Geometry: final body of the model. Coordinates: model frame, mm. A direction names the side the tool comes from. Round coordinates to 2 decimals unless told otherwise and drop trailing zeros. Write each loop counter-clockwise with the first axis right and the second up, starting at its lowest first coordinate (ties: lowest second). Pieces come first, ordered by that corner, then holes. Notation, with made-up numbers: M 14,69.25 L 34,69.25 A26 ccw 34,106.25 Z; hole C 40.25,-3 d3. An arc over 180 degrees is marked long. Answer as CSV lines item,"result". Start each with the question number.
Q1. First-contact query: pin 1 (1 mm diameter, centred on y = 1.5, z = 15.5, fed in from +X); pin 2 (2 mm diameter, centred on y = 3.5, z = 3, fed in from +X); pin 3 (6 mm diameter, centred on x = -30, z = 13, fed in from -Y). Flat tips, straight axial feed; report the tip coordinate or a pass-through.
Q2. Reachability of faces 1 (the flat face through (-8.507, 1.148, 4.405)), 2 (the flat face through (-7.088, 4.317, 13.477)), 3 (the flat face through (-7.07, 1.148, 12.973)) from +Z, -Z, +X, -X, +Y, -Y: full face, straight path, thin tool, end or side. Return the list, or none.
Q3. Section query C-C on y = -1.5. Output: boundary loops of the cut face in (x, z).
Q4. Section query A-A on x = -28.5. Output: boundary loops of the cut face in (y, z).
Q5. Section query B-B on y = 7.25. Output: boundary loops of the cut face in (x, z), and give its area (3 significant figures).
Q6. Ray query, probe 1 along Y at (x, z) = (-50.5, 15.25); probe 2 along X at (y, z) = (0.75, 11.75); probe 3 along Z at (x, y) = (-79, -1.5). Return the intervals inside material, ascending.
```python
from build123d import *

# Parameters (mm, degrees)
BOSS_EXTRUDE2_DEPTH      = 5.6
CHAMFER2_SIZE            = 2.328478482
CHAMFER2_SIZE_2          = 8.69
CHAMFER3_SIZE            = 8.69
CHAMFER3_SIZE_2          = 2.328478482
CHAMFER4_SIZE            = 8.69
CHAMFER4_SIZE_2          = 2.328478482
CHAMFER5_SIZE            = 8.69
CHAMFER5_SIZE_2          = 2.328478482
FILLET1_R                = 1
SKETCH8_R                = 6.42
BOSS_EXTRUDE3_DEPTH      = 58
FILLET2_R                = 3
CUT_EXTRUDE12_DEPTH      = 16
CUT_EXTRUDE13_DEPTH      = 119.774223563
CUT_EXTRUDE13_DEPTH_BACK = 119.774223563
SKETCH19_W               = 4.551969905
SKETCH19_H               = 31.016999287


with BuildPart() as part:
    # Sketch3 → Boss-Extrude2 (new body)
    with BuildSketch(Plane(origin=(0, 0, 0), x_dir=(1, 0, 0), z_dir=(0, 1, 0))):
        with BuildLine():
            Line((-55.958218902, 0), (34.866239796, 0))
            ThreePointArc((34.866239796, 0), (43.555159042, -8.688919246), (34.866239796, -17.377838493))
            Line((34.866239796, -17.377838493), (-55.633760204, -17.377838493))
            Line((-55.633760204, -17.377838493), (-59.133760204, -14.977838493))
            Line((-59.133760204, -14.977838493), (-59.132241437, -8.577838493))
            Line((-59.132241437, -8.577838493), (-59.132241437, -2.173298587))
            Line((-59.132241437, -2.173298587), (-55.958218902, 0))
        make_face()
    extrude(amount=BOSS_EXTRUDE2_DEPTH)

    # Chamfer2
    # the kernel refuses this chamfer: 8.69, 2.328478482 mm, written as the material it takes off along each edge
    with BuildSketch(Plane(origin=(57.431750241, 5.6, 17.377838493), x_dir=(0, -0.9905000388259545, 0.13751244702128881), z_dir=(-1, 0, 0))) as chamfer2_piece_1:
        Polygon((CHAMFER2_SIZE * 0.990500038922, -CHAMFER2_SIZE * 0.137512447035), (-CHAMFER2_SIZE_2 * 0.137512447021, -CHAMFER2_SIZE_2 * 0.990500038826), (0, 0), align=None)
    extrude(amount=135.63102089, mode=Mode.SUBTRACT)

    # Chamfer3
    # the kernel refuses this chamfer: 8.69, 2.328478482 mm, written as the material it takes off along each edge
    with BuildSketch(Plane(origin=(57.431750241, 0, 17.377838493), x_dir=(0, -0.009967146577156423, -0.9999503267608394), z_dir=(-1, 0, 0))) as chamfer3_piece_1:
        Polygon((CHAMFER3_SIZE * 0.999950326761, -CHAMFER3_SIZE * 0.00996714657716), (-CHAMFER3_SIZE_2 * 0.00996714657813, -CHAMFER3_SIZE_2 * 0.999950326858), (0, 0), align=None)
    extrude(amount=135.63102089, mode=Mode.SUBTRACT)

    # Chamfer4
    # the kernel refuses this chamfer: 8.69, 2.328478482 mm, written as the material it takes off along each edge
    with BuildSketch(Plane(origin=(-78.523729347, 5.6, 0), x_dir=(0, 0.00996714657715643, 0.9999503267608394), z_dir=(1, 0, 0))) as chamfer4_piece_1:
        Polygon((CHAMFER4_SIZE * 0.999950326761, CHAMFER4_SIZE * 0.00996714657716), (-CHAMFER4_SIZE_2 * 0.00996714657813, CHAMFER4_SIZE_2 * 0.999950326858), (0, 0), align=None)
    extrude(amount=135.955479588, mode=Mode.SUBTRACT)

    # Chamfer5
    # the kernel refuses this chamfer: 8.69, 2.328478482 mm, written as the material it takes off along each edge
    with BuildSketch(Plane(origin=(-78.523729347, 0, 0), x_dir=(0, -0.009967146577156423, 0.9999503267608394), z_dir=(1, 0, 0))) as chamfer5_piece_1:
        Polygon((CHAMFER5_SIZE * 0.999950326761, -CHAMFER5_SIZE * 0.00996714657716), (-CHAMFER5_SIZE_2 * 0.00996714657813, -CHAMFER5_SIZE_2 * 0.999950326858), (0, 0), align=None)
    extrude(amount=135.955479588, mode=Mode.SUBTRACT)

    # Fillet1
    fillet1_edges = [part.edges().sort_by_distance(p)[0] for p in [
        (-55.633760204, 2.8, 17.377838493),
    ]]
    fillet(fillet1_edges, radius=FILLET1_R)

    # Sketch8 → Boss-Extrude3 (add)
    with BuildSketch(Plane(origin=(-59.130202523, 0, -0.014032034), x_dir=(-0.00023730738394525297, 0, 0.9999999718426024), z_dir=(-0.9999999718426024, 0, -0.00023730738394525297))):
        with Locations(Location((8.591870769, 2.8, 0), (0, 0, 183.840787638))):
            Circle(SKETCH8_R)
    extrude(amount=BOSS_EXTRUDE3_DEPTH)

    # Fillet2
    fillet2_edges = [part.edges().sort_by_distance(p)[0] for p in [
        (-7.788554378, 5.599710413, 8.688919246),
    ]]
    fillet(fillet2_edges, radius=FILLET2_R)

    # Sketch16 → Cut-Extrude12 (cut)
    with BuildSketch(Plane.XY):
        Polygon((-58.943650552, 9.22), (-63.693726721, 9.22), (-58.943650552, 5.391659351), align=None)
        Polygon((-58.943650552, -3.62), (-63.693726721, -3.62), (-58.943650552, 0.208340649), align=None)
    extrude(amount=CUT_EXTRUDE12_DEPTH, mode=Mode.SUBTRACT)

    # Sketch19 → Cut-Extrude13 (cut, two sides: drawn at the far end of the back side and taken through both)
    with BuildSketch(Plane(origin=(0, 0, 0), x_dir=(1, 0, 0), z_dir=(0, 1, 0)).offset(-CUT_EXTRUDE13_DEPTH_BACK)):
        with Locations((-117.406701244, -5.968129835)):
            Rectangle(SKETCH19_W, SKETCH19_H)
    extrude(amount=CUT_EXTRUDE13_DEPTH + CUT_EXTRUDE13_DEPTH_BACK, mode=Mode.SUBTRACT)


solid = part.part
```
Entries:
1,pin 1,"stops at x = 40.79"
1,pin 2,"stops at x = 42.18"
1,pin 3,"stops at y = 0.35"
2,face 1,"-Z, +X, -Y"
2,face 2,"+Z, +X, +Y"
2,face 3,"+Z, +X, -Y"
3,outline,"M -115.13,3.8 L -61.06,3.81 L -61.06,13.34 L -115.13,13.33 Z"
4,outline,"M 0,8.69 L 2.33,0 L 3.27,0 L 5.39,7.91 A3 ccw 5.39,9.47 L 3.27,17.38 L 2.33,17.38 Z"
5,outline,"M -115.13,3.94 L -61.25,3.95 L -61.25,13.2 L -115.13,13.19 Z"
5,area,"499 mm^2"
6,probe 1,"y = 1.76 to 3.84"
6,probe 2,"x = -115.13 to -59.13"
6,probe 3,"z = 3.81 to 13.34"
